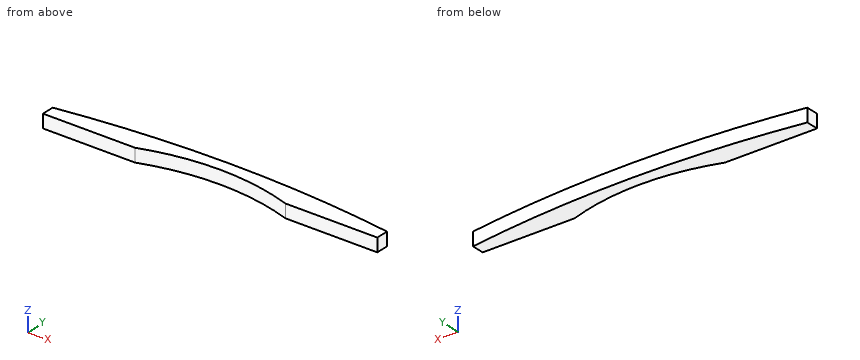
from build123d import *

# Parameters (mm, degrees)
BOSS_EXTRU_1_DEPTH = 8


with BuildPart() as part:
    # Esquisse1 → Boss.-Extru.1 (new body)
    with BuildSketch(Plane.XY):
        with BuildLine():
            Line((-100, 0), (-100, 7.5))
            ThreePointArc((-100, 7.5), (0, 15), (100, 7.5))
            Line((100, 7.5), (100, 0))
            Line((100, 0), (45, 0))
            ThreePointArc((45, 0), (0, 7.5), (-45, 0))
            Line((-45, 0), (-100, 0))
        make_face()
    extrude(amount=BOSS_EXTRU_1_DEPTH)


solid = part.part
The listing builds one solid part. Answer for the finished solid, in the listing's coordinates (mm). Give positions to 0.01 mm unless a question says otherwise; leave off trailing zeros. Order: outer loops, then holes, each group sorted by start corner. A loop starts at its lowest first (then second) coordinate and runs counter-clockwise, first axis right, second up. Notation, with made-up numbers: (-9, -40) - (22, -40) arc R30 cw to (22, -8) - close; hole circle Ø2 at (5.5, -16.75). An arc over 180 degrees is marked (long way). One line per item, written item: value. Start each with the question number.
1) Find the intervals of material crossed by L1, parallel to Y at x = -1, z = 2.25; L2, parallel to Y at x = -37, z = 4.25, in increasing order.
2) A cutting plane is placed at B-B on z = 1.5. Give the vertices of the cut face in (x, y), then the cut area to 3 significant figures.
3) A cutting plane is placed at C-C on x = -14.5. Give the vertices of the cut face in (y, z).
4) Given pin 1 Ø5 at (x, y) = (2.5, 10.5) entering from -Z; pin 2 Ø2 at (x, z) = (30, 4.5) entering from -Y, each flat-ended and moving along its own axis, determine where each tip first touches the part or whether it passes through.
5) A cutting plane is placed at A-A on y = 3.5. Give the vertices of the cut face in (x, z), then the cut area to 3 significant figures.
Answer sheet:
1. L1: y = 7.5 to 15
1. L2: y = 2.48 to 13.98
2. outline: (-100, 0) - (-45, 0) arc R138.75 cw to (45, 0) - (100, 0) - (100, 7.5) arc R670.42 ccw to (-100, 7.5) - close
2. area: 2,050 mm2
3. outline: (6.74, 0) - (14.84, 0) - (14.84, 8) - (6.74, 8) - close
4. pin 1: stops at z = 0
4. pin 2: stops at y = 3.99
5. outline: (-100, 0) - (-33.08, 0) - (-33.08, 8) - (-100, 8) - close; (33.08, 0) - (100, 0) - (100, 8) - (33.08, 8) - close
5. area: 1,070 mm2
